from build123d import *

# Parameters (mm, degrees)
EXTRUDE_1_DEPTH     = 4
EXTRUDE_START       = -2.2
SKETCH_2_W          = 15
SKETCH_2_H          = 4
EXTRUDE_2_DEPTH     = 0.8
SKETCH_3_R          = 0.5
EXTRUDE_3_DEPTH     = 1
FILLET_1_R          = 0.5
SKETCH_4_R          = 0.4
EXTRUDE_4_DEPTH     = 1.75
CUT_EXTRUDE_START   = 1.75
CUT_EXTRUDE_1_DEPTH = 1.75
SKETCH_8_R          = 0.5
CUT_EXTRUDE_2_DEPTH = 0.1


with BuildPart() as part:
    # 草图1 → 凸台-拉伸1 (new body)
    with BuildSketch(Plane.XY):
        with BuildLine():
            Line((0, 2), (11, 2))
            ThreePointArc((11, 2), (13, 0), (11, -2))
            Line((11, -2), (0, -2))
            ThreePointArc((0, -2), (-2, 0), (0, 2))
        make_face()
    extrude(amount=EXTRUDE_1_DEPTH)

    # 草图2 → 凸台-拉伸2 (add)
    with BuildSketch(Plane(origin=(0, 0, 0), x_dir=(-1, 0, 0), z_dir=(0, 0, -1)).offset(EXTRUDE_START)):
        with Locations((-5.5, 0)):
            Rectangle(SKETCH_2_W, SKETCH_2_H)
    extrude(amount=-EXTRUDE_2_DEPTH)

    # 草图3 → 凸台-拉伸3 (add)
    with BuildSketch(Plane(origin=(0, 0, 0), x_dir=(-1, 0, 0), z_dir=(0, 0, -1))):
        with Locations(Location((-8.04, 0, 0), (0, 0, 180))):
            Circle(SKETCH_3_R)
        with Locations(Location((-5.5, 0, 0), (0, 0, 180))):
            Circle(SKETCH_3_R)
        with Locations(Location((-2.96, 0, 0), (0, 0, 180))):
            Circle(SKETCH_3_R)
    extrude(amount=EXTRUDE_3_DEPTH)

    # 圆角1
    fillet_1_edges = [part.edges().sort_by_distance(p)[0] for p in [
        (7.54, 0, -1),
        (5, 0, -1),
        (2.46, 0, -1),
    ]]
    fillet(fillet_1_edges, radius=FILLET_1_R)

    # 草图4 → 凸台-拉伸4 (add)
    with BuildSketch(Plane.XY.offset(4)):
        with Locations((2.96, 0)):
            Circle(SKETCH_4_R)
        with Locations((5.5, 0)):
            Circle(SKETCH_4_R)
        with Locations((8.04, 0)):
            Circle(SKETCH_4_R)
    extrude(amount=EXTRUDE_4_DEPTH)

    # 草图7 → 切除-拉伸1 (cut)
    with BuildSketch(Plane(origin=(0, 0, 0), x_dir=(-1, 0, 0), z_dir=(0, 0, -1)).offset(CUT_EXTRUDE_START)):
        with BuildLine():
            Line((0, 2), (-11, 2))
            ThreePointArc((-11, 2), (-13, 0), (-11, -2))
            Line((-11, -2), (0, -2))
            ThreePointArc((0, -2), (2, 0), (0, 2))
        make_face()
    extrude(amount=-CUT_EXTRUDE_1_DEPTH, mode=Mode.SUBTRACT)

    # 草图8 → 切除-拉伸2 (cut)
    with BuildSketch(Plane(origin=(0, 0, 0), x_dir=(-1, 0, 0), z_dir=(0, 0, -1))):
        with Locations((-8.04, 0)):
            Circle(SKETCH_8_R)
        with Locations((-5.5, 0)):
            Circle(SKETCH_8_R)
        with Locations((-2.96, 0)):
            Circle(SKETCH_8_R)
    extrude(amount=-CUT_EXTRUDE_2_DEPTH, mode=Mode.SUBTRACT)


solid = part.part
Can you work these out from the model? Positions are in its coordinate system, mm. A direction names the side the tool comes from. Give positions to 0.01 mm unless a question says otherwise; leave off trailing zeros. Order: outer loops, then holes, each group sorted by start corner. A loop starts at its lowest first (then second) coordinate and runs counter-clockwise, first axis right, second up. Notation, with made-up numbers: M 66,70 L 75,70 A23 ccw 75,98 Z; hole C 27.25,78.25 d3. An arc over 180 degrees is marked long. Use one line per item in the form item = value. Start each with the question number.
Item 1: If we section it at C-C (z = 5.2): Write out the boundary of the cut face in (x, y), then the cut area to 3 significant figures.
Item 2: For faces 1 (the cylindrical face through (-2, 0, 3.5)), 2 (the flat face through (12.6, -1.5, 3)), 3 (the cylindrical face through (5.88, 0.12, 4.86)), which set-ups out of +Z, -Z, +X, -X, +Y, -Y let a thin tool reach every point of the face, with its end or its side?
Item 3: Will these pins go through, and if not, where does the flat tip stop? pin 1 Ø1.1 at (x, y) = (5.5, 0) entering from -Z; pin 2 Ø0.8 at (x, y) = (3, 0) entering from -Z; pin 3 Ø1 at (x, y) = (-1, 1) entering from +Z.
Item 4: We'd pull the mould along Y, two halves only. Please class faces 4 (the flat face through (-1.5, 1.6, 2.2)), 5 (the flat face through (3, 0, 0.1)), 6 (the flat face through (6, 2, 2)): +Y half, -Y half, draft (parallel to the pull), parting line (faces both ways), or undercut.
Item 5: If we section it at A-A (y = -1.2): Write out the boundary of the cut face in (x, z).
Item 6: If I drill on line 1 along Y through (x, z) = (8.04, 0.05); line 2 along Z through (x, y) = (8, -0.05); line 3 along Z through (x, y) = (8.5, 0.35), over which ranges is the centre line in solid material (lowest first)?
Item 7: If we section it at B-B (x = 2.96): Write out the boundary of the cut face in (y, z).
Item 8: If we section it at D-D (z = 0.5): Write out the boundary of the cut face in (x, y).
Outcome:
q1.outline = C 2.96,0 d0.8; C 5.5,0 d0.8; C 8.04,0 d0.8
q1.area = 1.51 mm2
q2.face_1 = +Z, -X
q2.face_2 = +Z, +X, -Y
q2.face_3 = +Z
q3.pin_1 = 0
q3.pin_2 = 0.1
q3.pin_3 = 4
q4.face_4 = draft
q4.face_5 = undercut
q4.face_6 = +Y half
q5.outline = M -2,2.2 L -1.6,2.2 L -1.6,0 L 12.6,0 L 12.6,2.2 L 13,2.2 L 13,3 L 12.6,3 L 12.6,4 L -1.6,4 L -1.6,3 L -2,3 Z
q6.line_1 = -2 to -0.5, 0.5 to 2
q6.line_2 = 0.1 to 5.75
q6.line_3 = 0 to 4
q7.outline = M -2,0 L -0.5,0 L -0.5,0.1 L 0.5,0.1 L 0.5,0 L 2,0 L 2,4 L 0.4,4 L 0.4,5.75 L -0.4,5.75 L -0.4,4 L -2,4 Z
q8.outline = M 0,-2 L 11,-2 A2 ccw 11,2 L 0,2 A2 ccw Z
